Geometry: final body of the model. Coordinates: model frame, mm. A direction names the side the tool comes from. Round coordinates to 2 decimals unless told otherwise and drop trailing zeros. Write each loop counter-clockwise with the first axis right and the second up, starting at its lowest first coordinate (ties: lowest second). Pieces come first, ordered by that corner, then holes. Notation, with made-up numbers: M -29,13.5 L 9,13.5 A12 ccw 9,26.5 Z; hole C -36,-1 d8. An arc over 180 degrees is marked long. Put each result on its own line as item: value. Start each with the question number.
```python
from build123d import *

# Parameters (mm, degrees)
SKETCH2_W                         = 18
SKETCH2_H                         = 22
SKETCH2_W_2                       = 4
BOSS_EXTRUDE1_DEPTH               = 4
SKETCH2_4_W                       = 18
SKETCH2_4_H                       = 10.1
SKETCH2_4_W_2                     = 6
SKETCH2_4_H_2                     = 2.1
BOSS_EXTRUDE2_DEPTH               = 12
SKETCH2_5_W                       = 4
SKETCH2_5_H                       = 22
BOSS_EXTRUDE3_DEPTH               = 20
F_3_2_3_2_MOUNT_HOLES_D           = 3.2
F_3_2_3_2_MOUNT_HOLES_ON_FACE_2_D = 3.2
F_3_2_3_2_MOUNT_HOLES_ON_FACE_3_D = 3.2
FILLET2_R                         = 6
FILLET1_R                         = 2
FILLET3_R                         = 4


with BuildPart() as part:
    # Sketch2 → Boss-Extrude1 (new body)
    with BuildSketch(Plane(origin=(0, 0, 0), x_dir=(1, 0, 0), z_dir=(0, 1, 0))):
        with Locations((0, 11)):
            Rectangle(SKETCH2_W, SKETCH2_H)
        with Locations((11, 11)):
            Rectangle(SKETCH2_W_2, SKETCH2_H)
    extrude(amount=BOSS_EXTRUDE1_DEPTH)

    # Sketch2<4> → Boss-Extrude2 (add)
    with BuildSketch(Plane(origin=(0, 0, 0), x_dir=(1, 0, 0), z_dir=(0, 1, 0))):
        with Locations((0, 5.05)):
            Rectangle(SKETCH2_4_W, SKETCH2_4_H)
        with Locations((0, 5.05)):
            Rectangle(SKETCH2_4_W_2, SKETCH2_4_H_2, mode=Mode.SUBTRACT)
    extrude(amount=BOSS_EXTRUDE2_DEPTH)

    # Sketch2<5> → Boss-Extrude3 (add)
    with BuildSketch(Plane(origin=(0, 0, 0), x_dir=(1, 0, 0), z_dir=(0, 1, 0))):
        with Locations((11, 11)):
            Rectangle(SKETCH2_5_W, SKETCH2_5_H)
    extrude(amount=BOSS_EXTRUDE3_DEPTH)

    # Ø3.2 (3.2) Mount Holes (through all)
    with Locations(Plane(origin=(0, 7.4, 0), x_dir=(1, 0, 0), z_dir=(0, 0, 1))):
        with Locations((0, 0)):
            Hole(F_3_2_3_2_MOUNT_HOLES_D / 2)

    # Ø3.2 (3.2) Mount Holes on face 2 (through all)
    with Locations(Plane(origin=(0, 0, -16), x_dir=(0, 0, -1), z_dir=(0, -1, 0))):
        with Locations((0, 0)):
            Hole(F_3_2_3_2_MOUNT_HOLES_ON_FACE_2_D / 2)

    # Ø3.2 (3.2) Mount Holes on face 3 (through all)
    with Locations(Plane(origin=(13, 13, -16), x_dir=(0, 0, 1), z_dir=(1, 0, 0))):
        with Locations((0, 0)):
            Hole(F_3_2_3_2_MOUNT_HOLES_ON_FACE_3_D / 2)

    # Fillet2
    fillet2_edges = [part.edges().sort_by_distance(p)[0] for p in [
        (9, 12, -5.05),
    ]]
    fillet(fillet2_edges, radius=FILLET2_R - 0.0001)  # a hair under: the kernel refuses the full size

    # Fillet1
    fillet1_edges = [part.edges().sort_by_distance(p)[0] for p in [
        (9, 10.99995, -10.1),
        (0, 4, -10.1),
        (9, 4, -16.05),
    ]]
    fillet(fillet1_edges, radius=FILLET1_R)

    # Fillet3
    fillet3_edges = [part.edges().sort_by_distance(p)[0] for p in [
        (-9, 12, -5.05),
        (11, 20, -22),
        (-9, 2, -22),
    ]]
    fillet(fillet3_edges, radius=FILLET3_R)


solid = part.part
```
1) Section D-D, the plane z = -13.25. Output: boundary loops of the cut face in (x, y), and give its area (3 significant figures).
2) First-contact query: pin 1 (3 mm diameter, centred on x = 0, y = 7.4, fed in from +Z); pin 2 (2.5 mm diameter, centred on x = -3.5, y = 9.5, fed in from -Z); pin 3 (5 mm diameter, centred on x = 0, z = -16, fed in from +Y); pin 4 (1 mm diameter, centred on y = 9.5, z = -10, fed in from -X). Flat tips, straight axial feed; report the tip coordinate or a pass-through.
3) Section A-A, the plane z = -16. Output: boundary loops of the cut face in (x, y).
4) Section B-B, the plane y = 13. Output: boundary loops of the cut face in (x, z).
5) Section C-C, the plane z = -8.75. Output: boundary loops of the cut face in (x, y).
6) Access query for faces 4 (the face through (4, 8, 0)), 5 (the face through (3.84, 4.6, -10.67)), 6 (the face through (0, 4, -5)). Directions: +Z, -Z, +X, -X, +Y, -Y. A direction counts if a zero-diameter tool reaches every point of the face in a straight line with its end or side. Return the directions, or none.
7) Draft query along X for faces 1 (the face through (-1, 4, -18)), 2 (the face through (-7.797, 10.859, -5.121)), 3 (the face through (0.35, 5.84, -8.13)). Return one class per face: +X half, -X half, draft (parallel to the pull), parting line (faces both ways), or undercut.
8) Ray query, probe 1 along X at (y, z) = (7.5, -3); probe 2 along Y at (x, z) = (10.55, -16); probe 3 along Z at (x, y) = (5, 10). Return the intervals inside material, ascending.
Solved:
1. outline: M -9,0 L 13,0 L 13,20 L 9,20 L 9,6 A2 cw 7,4 L -9,4 Z
1. area: 153 mm2
2. pin 1: passes through
2. pin 2: stops at z = -10.1
2. pin 3: stops at y = 4
2. pin 4: stops at x = -8.87
3. outline: M -9,0 L -1.6,0 L -1.6,4 L -9,4 Z; M 1.6,0 L 13,0 L 13,11.4 L 9,11.4 L 9,6 A2 cw 7,4 L 1.6,4 Z; M 9,14.6 L 13,14.6 L 13,20 L 9,20 Z
4. outline: M 6.32,-10.1 L 7,-10.1 A2 cw 9,-12.1 L 9,-14.4 L 13,-14.4 L 13,0 L 6.32,0 Z; M 9,-22 L 13,-22 L 13,-17.6 L 9,-17.6 Z
5. outline: M -9,0 L 13,0 L 13,20 L 9,20 L 9,18 A6 cw 3,12 L -5,12 A4 ccw -9,8 Z; hole C 0,7.4 d3.2
6. face 4: +Z, +X, -X, +Y, -Y
6. face 5: -Z, -X, +Y
6. face 6: +Y
7. face 1: draft
7. face 2: -X half
7. face 3: undercut
8. probe 1: x = -9 to -1.6, 1.6 to 13
8. probe 2: y = 0 to 11.4, 14.6 to 20
8. probe 3: z = -10.1 to 0
